Here's how the part is built. I have some questions about the finished solid (model axes, mm). A direction names the side the tool comes from. Coordinates: 2 decimals unless noted, no trailing zeros. Order: outer loops, then holes, each group sorted by start corner. A loop starts at its lowest first (then second) coordinate and runs counter-clockwise, first axis right, second up. Notation, with made-up numbers: (-29.75, 4.5) - (11.25, 4.5) arc R27 cw to (11.25, 40.5) - close; hole circle Ø6 at (-6, 46.5). An arc over 180 degrees is marked (long way). Answer in a Markdown table with one row per item. Add a question column.
Item 1: I want a section at B-B (z = 9). Please give me the cut outline in (x, y), plus the area to 3 significant figures.
Item 2: I want a section at A-A (y = 0). Please give me the cut outline in (x, z).
Item 3: I want a section at D-D (z = 22.25). Please give me the cut outline in (x, y), plus the area to 3 significant figures.
Item 4: On a 3-axis mill with a long thin cutter (end or side, diameter ignored), from which of +Z, -Z, +X, -X, +Y, -Y can I reach the whole of each face in a straight line? I mean faces 1 (the flat face through (-42.91, 0, 19)), 2 (the flat face through (-11, 20.2, 10)), 3 (the flat face through (-32, 22.702, 10)), 4 (the flat face through (-17, 0, 0)), 5 (the flat face through (-11, -20.2, 10)). Say none if no direction works.
Item 5: If I drill on line 1 along Z through (x, y) = (3, -11.5); line 2 along X through (y, z) = (-1, 14.75); line 3 along Z through (x, y) = (-33, -26), over which ranges is the centre line in solid material (lowest first)? Write a range as from..to.
Item 6: Thinking about a two-plate mould opening in X: for faces 6 (the flat face through (-36, 0, 20)), 7 (the flat face through (-42.91, 31, 19)), 8 (the cylindrical face through (-42.88, -25.56, 23.7)), 9 (the flat face through (-40, 31, 17)), which applies, +X half, -X half, draft (parallel to the pull), parting line (faces both ways), or undercut?
Item 7: Will these pins go through, and if not, where does the flat tip stop? pin 1 Ø0.7 at (y, z) = (32, 18) entering from +X; pin 2 Ø4 at (x, z) = (3, 5.5) entering from -Y; pin 3 Ø4 at (x, y) = (12, 2.5) entering from +Z.
Item 8: I want a section at C-C (x = 4). Please give me the cut outline in (y, z).
```python
from build123d import *

# Parameters (mm, degrees)
SKETCH_2_R          = 11.1
EXTRUDE_4_DEPTH     = 20
CUT_EXTRUDE_1_DEPTH = 10
EXTRUDE_5_DEPTH     = 3
EXTRUDE_6_DEPTH     = 7.5
SKETCH_19_R         = 2.85
CUT_EXTRUDE_2_DEPTH = 10
EXTRUDE_7_DEPTH     = 3


with BuildPart() as part:
    # Эскиз2 → Бобышка-Вытянуть4 (new body)
    with BuildSketch(Plane.XY):
        with BuildLine():
            Line((0, 20.2), (-22.659630228, 20.2))
            Line((-22.659630228, 20.2), (-22.659630228, 32.623416793))
            Line((-22.659630228, 32.623416793), (-30.159630228, 32.623416793))
            Line((-30.159630228, 32.623416793), (-30.159630228, -32.623416793))
            Line((-30.159630228, -32.623416793), (-22.659630228, -32.623416793))
            Line((-22.659630228, -32.623416793), (-22.659630228, -20.2))
            Line((-22.659630228, -20.2), (0, -20.2))
            ThreePointArc((0, -20.2), (20.2, 0), (0, 20.2))
        make_face()
        Circle(SKETCH_2_R, mode=Mode.SUBTRACT)
    extrude(amount=EXTRUDE_4_DEPTH)

    # Эскиз8 → Вырез-Вытянуть1 (cut)
    with BuildSketch(Plane(origin=(-22.659630228, 0, 0), x_dir=(0, 0, -1), z_dir=(1, 0, 0))):
        with BuildLine():
            ThreePointArc((-10, -23.561708397), (-12.85, -26.411708397), (-10, -29.261708397))
            Line((-10, -29.261708397), (-10, -23.561708397))
        make_face()
        with BuildLine():
            Line((-10, -23.561708397), (-10, -29.261708397))
            ThreePointArc((-10, -29.261708397), (-7.984745674, -28.426962723), (-7.15, -26.411708397))
            ThreePointArc((-7.15, -26.411708397), (-7.984745674, -24.39645407), (-10, -23.561708397))
        make_face()
        with BuildLine():
            ThreePointArc((-7.15, 26.411708397), (-7.984745674, 28.426962723), (-10, 29.261708397))
            Line((-10, 29.261708397), (-10, 23.561708397))
            ThreePointArc((-10, 23.561708397), (-7.984745674, 24.39645407), (-7.15, 26.411708397))
        make_face()
        with BuildLine():
            Line((-10, 23.561708397), (-10, 29.261708397))
            ThreePointArc((-10, 29.261708397), (-12.85, 26.411708397), (-10, 23.561708397))
        make_face()
    extrude(amount=-CUT_EXTRUDE_1_DEPTH, mode=Mode.SUBTRACT)

    # Эскиз15 → Бобышка-Вытянуть5 (add)
    with BuildSketch(Plane.ZY.offset(30.159630228)):
        Polygon((7.25, 22.701708397), (10, 22.701708397), (12.75, 22.701708397), (12.75, -22.701708397), (7.25, -22.701708397), align=None)
        Polygon((7.25, 32.623416793), (7.25, 30.121708397), (10, 30.121708397), (12.75, 30.121708397), (12.75, 32.623416793), align=None)
        Polygon((10, -30.121708397), (7.756029521, -30.121708397), (7.25, -30.121708397), (7.25, -32.623416793), (12.75, -32.623416793), (12.75, -30.121708397), align=None)
    extrude(amount=EXTRUDE_5_DEPTH)

    # Эскиз18 → Бобышка-Вытянуть6 (add)
    with BuildSketch(Plane.XY.offset(20)):
        Polygon((-30.159630228, -32.623416793), (-50.159630228, -32.623416793), (-50.159630228, 32.623416793), (-30.159630228, 32.623416793), (-22.659630228, 32.623416793), (-22.659630228, -32.623416793), align=None)
    extrude(amount=EXTRUDE_6_DEPTH)

    # Эскиз19 → Вырез-Вытянуть2 (cut)
    with BuildSketch(Plane(origin=(0, 0, 20), x_dir=(-1, 0, 0), z_dir=(0, 0, -1))):
        with Locations((40.159630228, -26.413416793)):
            Circle(SKETCH_19_R)
        with BuildLine():
            Line((37.409630228, 27.161748271), (37.409630228, 25.665085316))
            ThreePointArc((37.409630228, 25.665085316), (40.159630228, 23.563416793), (42.909630228, 25.665085316))
            Line((42.909630228, 25.665085316), (42.909630228, 27.161748271))
            ThreePointArc((42.909630228, 27.161748271), (40.159630228, 29.263416793), (37.409630228, 27.161748271))
        make_face()
    extrude(amount=-CUT_EXTRUDE_2_DEPTH, mode=Mode.SUBTRACT)

    # Эскиз19<14> → Бобышка-Вытянуть7 (add)
    with BuildSketch(Plane(origin=(0, 0, 20), x_dir=(-1, 0, 0), z_dir=(0, 0, -1))):
        Polygon((37.409630228, -22.703416793), (40.159630228, -22.703416793), (42.909630228, -22.703416793), (42.909630228, 22.703416793), (40.159630228, 22.703416793), (37.409630228, 22.703416793), align=None)
        Polygon((37.409630228, 32.623416793), (37.409630228, 30.123416793), (40.159630228, 30.123416793), (42.909630228, 30.123416793), (42.909630228, 32.623416793), align=None)
        Polygon((42.909630228, -30.123416793), (40.159630228, -30.123416793), (37.409630228, -30.123416793), (37.409630228, -32.623416793), (42.909630228, -32.623416793), align=None)
    extrude(amount=EXTRUDE_7_DEPTH)


solid = part.part
```
Values follow:
| question | item | result |
|---|---|---|
| 1 | outline | (-33.16, -32.62) - (-22.66, -32.62) - (-22.66, -29.08) - (-30.16, -29.08) - (-30.16, -30.12) - (-33.16, -30.12) - close; (-33.16, -22.7) - (-30.16, -22.7) - (-30.16, -23.74) - (-22.66, -23.74) - (-22.66, -20.2) - (0, -20.2) arc R20.2 ccw to (0, 20.2) - (-22.66, 20.2) - (-22.66, 23.74) - (-30.16, 23.74) - (-30.16, 22.7) - (-33.16, 22.7) - close; (-33.16, 30.12) - (-30.16, 30.12) - (-30.16, 29.08) - (-22.66, 29.08) - (-22.66, 32.62) - (-33.16, 32.62) - close; hole circle Ø22.2 at (0, 0) |
| 1 | area | 1,730 mm^2 |
| 2 | outline | (-50.16, 20) - (-42.91, 20) - (-42.91, 17) - (-37.41, 17) - (-37.41, 20) - (-30.16, 20) - (-30.16, 12.75) - (-33.16, 12.75) - (-33.16, 7.25) - (-30.16, 7.25) - (-30.16, 0) - (-11.1, 0) - (-11.1, 20) - (-22.66, 20) - (-22.66, 27.5) - (-50.16, 27.5) - close; (11.1, 0) - (20.2, 0) - (20.2, 20) - (11.1, 20) - close |
| 3 | outline | (-50.16, -32.62) - (-22.66, -32.62) - (-22.66, 32.62) - (-50.16, 32.62) - close; hole circle Ø5.7 at (-40.16, -26.41); hole (-42.91, 25.67) arc R2.85 ccw to (-37.41, 25.67) - (-37.41, 27.16) arc R2.85 ccw to (-42.91, 27.16) - close |
| 3 | area | 1,740 mm^2 |
| 4 | face 1 | -Z, -X, +Y, -Y |
| 4 | face 2 | +Z, -Z, +X, +Y |
| 4 | face 3 | -Z, -X |
| 4 | face 4 | -Z, +X, -X, +Y, -Y |
| 4 | face 5 | +Z, -Z, +X, -Y |
| 5 | line 1 | z = 0..20 |
| 5 | line 2 | x = -30.16..-11.05, 11.05..20.18 |
| 5 | line 3 | z = 20..27.5 |
| 6 | face 6 | undercut |
| 6 | face 7 | -X half |
| 6 | face 8 | undercut |
| 6 | face 9 | draft |
| 7 | pin 1 | stops at x = -22.66 |
| 7 | pin 2 | stops at y = -20.18 |
| 7 | pin 3 | stops at z = 20 |
| 8 | outline | (-19.8, 0) - (-10.35, 0) - (-10.35, 20) - (-19.8, 20) - close; (10.35, 0) - (19.8, 0) - (19.8, 20) - (10.35, 20) - close |
